The model under review builds one solid part; all positions refer to its coordinate system, in mm. Face numbers are marked on the shaded views. A direction names the side the tool comes from. Coordinates: 2 decimals unless noted, no trailing zeros. Loops run counter-clockwise (first coordinate to the right, second up) from the corner with the lowest first, then second, coordinate; pieces in that order, holes last. Notation, with made-up numbers: (51, 7) - (55, 7) arc R14 cw to (55, 24) - close; hole circle Ø6 at (28, 77). An arc over 180 degrees is marked (long way). Use a Markdown table: item, result. Add a question column.
1) The part is to be moulded in two halves that separate along Y. For the marked faces 1, 2 and 3, say which applies: pulls with the +Y half, pulls with the -Y half, needs draft (parallel to the pull), parting line crosses it, or undercut.
2) Add section B-B, the plane y = -25. Give the boundary of the cut face in (x, z).
3) Add section D-D, the plane x = 23.5. Give the boundary of the cut face in (y, z), and give its area (3 significant figures).
4) Add section A-A, the plane y = 20. Give the boundary of the cut face in (x, z).
5) To check wall thickness, follow L1, parallel to Y at x = 9, z = -18.05; L2, parallel to Y at x = 3, z = 10; L3, parallel to Z at x = 18, y = 28.5. State the ranges of each line that lie inside material, in increasing order. Write a range as [from, to].
6) For the marked faces 4, 5, 6, 7 and 8, list the 3-axis set-ups (+Z, -Z, +X, -X, +Y, -Y) from which the entire face can be reached by the end or side of a thin tool; tool diameter is ignored.
7) Clearance check with flat-ended pins moving along their axes: pin 1 (3 mm diameter, centred on x = 16, z = 0, fed in from -Y); pin 2 (2.5 mm diameter, centred on x = 9, y = -16, fed in from +Z); pin 3 (6 mm diameter, centred on y = -14.5, z = -8, fed in from +X); pin 4 (10 mm diameter, centred on y = -1.5, z = -6.5, fed in from -X). State where each tip first meets the part, or that it passes through.
8) Add section C-C, the plane x = 16. Give the boundary of the cut face in (y, z).
```python
from build123d import *

# Parameters (mm, degrees)
SKETCH1_W           = 38
SKETCH1_H           = 64
SKETCH1_W_2         = 34
SKETCH1_H_2         = 60
BOSS_EXTRUDE1_DEPTH = 32
SKETCH2_R           = 1.5
CUT_EXTRUDE1_DEPTH  = 60.093146811
BOSS_EXTRUDE3_REACH = 74.312
SKETCH7_R           = 16
SKETCH8_R           = 2.5
CUT_EXTRUDE2_DEPTH  = 75.033776076
SKETCH9_R           = 6
CUT_EXTRUDE3_DEPTH  = 40


with BuildPart() as part:
    # Sketch1 → Boss-Extrude1 (new body)
    with BuildSketch(Plane(origin=(0, 0, 0), x_dir=(0, 0, -1), z_dir=(1, 0, 0))):
        Rectangle(SKETCH1_W, SKETCH1_H)
        Rectangle(SKETCH1_W_2, SKETCH1_H_2, mode=Mode.SUBTRACT)
    extrude(amount=BOSS_EXTRUDE1_DEPTH)

    # Sketch2 → Cut-Extrude1 (cut, through all)
    with BuildSketch(Plane.XY.offset(19)):
        with Locations((9, 20)):
            Circle(SKETCH2_R)
        with Locations((23, 20)):
            Circle(SKETCH2_R)
        with Locations((16, 1.663521733)):
            Circle(SKETCH2_R)
        with Locations((9, -16)):
            Circle(SKETCH2_R)
        with Locations((23, -16)):
            Circle(SKETCH2_R)
    extrude(amount=-CUT_EXTRUDE1_DEPTH, mode=Mode.SUBTRACT)

    # Sketch7 → Boss-Extrude3 (add, up to next)
    with BuildSketch(Plane(origin=(0, -30, 0), x_dir=(1, 0, 0), z_dir=(0, 1, 0)), mode=Mode.PRIVATE) as boss_extrude3_sk1:
        with Locations(Location((16, 0, 0), (0, 0, 180))):
            Circle(SKETCH7_R)
    boss_extrude3_tool1 = extrude(boss_extrude3_sk1.sketch, amount=BOSS_EXTRUDE3_REACH, mode=Mode.PRIVATE) - part.part
    add(boss_extrude3_tool1.solids().sort_by_distance((16, -30, 0))[0])

    # Sketch8 → Cut-Extrude2 (cut, through all)
    with BuildSketch(Plane(origin=(0, 32, 0), x_dir=(1, 0, 0), z_dir=(0, 1, 0))):
        with Locations(Location((16, 0, 0), (0, 0, 270))):
            Circle(SKETCH8_R)
    extrude(amount=-CUT_EXTRUDE2_DEPTH, mode=Mode.SUBTRACT)

    # Sketch9 → Cut-Extrude3 (cut)
    with BuildSketch(Plane.XZ.offset(32)):
        with Locations(Location((16, 0, 0), (0, 0, 270))):
            Circle(SKETCH9_R)
    extrude(amount=-CUT_EXTRUDE3_DEPTH, mode=Mode.SUBTRACT)


solid = part.part
```
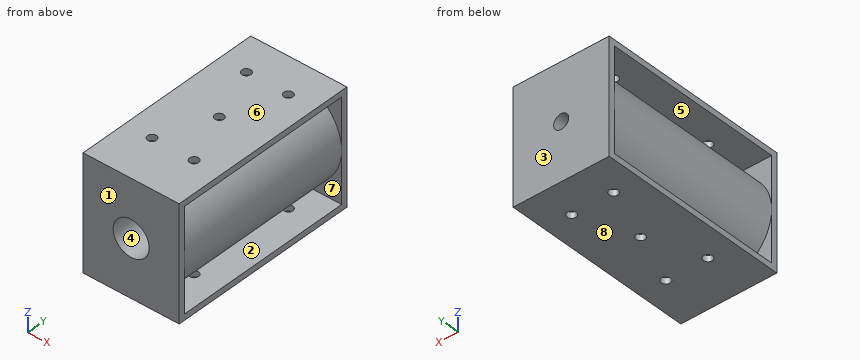
From the geometry:
| question | item | result |
|---|---|---|
| 1 | face 1 | pulls with the -Y half |
| 1 | face 2 | undercut |
| 1 | face 3 | pulls with the +Y half |
| 2 | outline | (0, -19) - (32, -19) - (32, -17) - (0, -17) - close; circle Ø32 at (16, 0); (0, 17) - (32, 17) - (32, 19) - (0, 19) - close; hole circle Ø12 at (16, 0) |
| 3 | outline | (-32, -19) - (-17.41, -19) - (-17.41, -17) - (-30, -17) - (-30, -14.13) - (30, -14.13) - (30, -17) - (21.41, -17) - (21.41, -19) - (32, -19) - (32, 19) - (21.41, 19) - (21.41, 17) - (30, 17) - (30, 14.13) - (-30, 14.13) - (-30, 17) - (-17.41, 17) - (-17.41, 19) - (-32, 19) - close; (-14.59, -19) - (18.59, -19) - (18.59, -17) - (-14.59, -17) - close; (-14.59, 17) - (18.59, 17) - (18.59, 19) - (-14.59, 19) - close |
| 3 | area | 2,070 mm^2 |
| 4 | outline | (0, -19) - (7.5, -19) - (7.5, -17) - (0, -17) - close; circle Ø32 at (16, 0); (0, 17) - (7.5, 17) - (7.5, 19) - (0, 19) - close; (10.5, -19) - (21.5, -19) - (21.5, -17) - (10.5, -17) - close; (10.5, 17) - (21.5, 17) - (21.5, 19) - (10.5, 19) - close; (24.5, -19) - (32, -19) - (32, -17) - (24.5, -17) - close; (24.5, 17) - (32, 17) - (32, 19) - (24.5, 19) - close; hole circle Ø5 at (16, 0) |
| 5 | L1 | y = [-32, -17.5], [-14.5, 18.5], [21.5, 32] |
| 5 | L2 | y = [-32, -30], [30, 32] |
| 5 | L3 | z = [-19, -17], [-15.87, -1.5], [1.5, 15.87], [17, 19] |
| 6 | face 4 | -Y |
| 6 | face 5 | +X, -X |
| 6 | face 6 | +Z, +X, -X, +Y, -Y |
| 6 | face 7 | none |
| 6 | face 8 | -Z, +X, -X, +Y, -Y |
| 7 | pin 1 | passes through |
| 7 | pin 2 | stops at z = 14.93 |
| 7 | pin 3 | stops at x = 31.2 |
| 7 | pin 4 | stops at x = 0.07 |
| 8 | outline | (-32, -19) - (0.16, -19) - (0.16, -17) - (-30, -17) - (-30, -16) - (30, -16) - (30, -17) - (3.16, -17) - (3.16, -19) - (32, -19) - (32, -2.5) - (8, -2.5) - (8, -6) - (-32, -6) - close; (-32, 6) - (8, 6) - (8, 2.5) - (32, 2.5) - (32, 19) - (3.16, 19) - (3.16, 17) - (30, 17) - (30, 16) - (-30, 16) - (-30, 17) - (0.16, 17) - (0.16, 19) - (-32, 19) - close |
